Verification items for this drawing (mm, ordinates from the low corner). Coordinates: 2 decimals unless noted, no trailing zeros. Write each loop counter-clockwise with the first axis right and the second up, starting at its lowest first coordinate (ties: lowest second). Pieces come first, ordered by that corner, then holes. Notation, with made-up numbers: M 64,72 L 80,72 A17 cw 80,82 Z; hole C 23.25,71.25 d9. An arc over 180 degrees is marked long. Answer as CSV lines item,"result". Start each with the question number.
1) Material ranges on L1, parallel to Y at x = 7.75, z = 19.05 (1 decimal); L2, parallel to Z at x = 9.5, y = 11.5 (1 decimal); L3, parallel to Z at x = 11.5, y = 19.05 (1 decimal), recorded low to high. Write a range as [from, to].
2) Section check B-B (y = 19.05). Record the cut outline in (x, z) (1 decimal).
3) Draft check along Y on the marked faces 1, 2 and 3. Enter one of: +Y half, -Y half, draft (parallel to the pull), parting line (faces both ways), or undercut.
4) Go/stop test with flat-tipped pins: pin 1 Ø10 at (y, z) = (13.97, 10.25) entering from +X; pin 2 Ø5.5 at (y, z) = (13.97, 27.85) entering from +X; pin 3 Ø3 at (x, z) = (4.5, 33) entering from -Y; pin 4 Ø5 at (x, y) = (9, 32.5) entering from +Z (1 decimal). Record where each tip stops, or that it passes through.
5) Section check A-A (z = 19.05). Record the cut outline in (x, y) (1 decimal).
6) Section check C-C (x = 8). State how many separate pieces and enclosed holes the cut face has, and give its area (3 significant figures).
7) Section check D-D (y = 13.97). Record the cut outline in (x, z) (1 decimal), and give its area (3 significant figures).
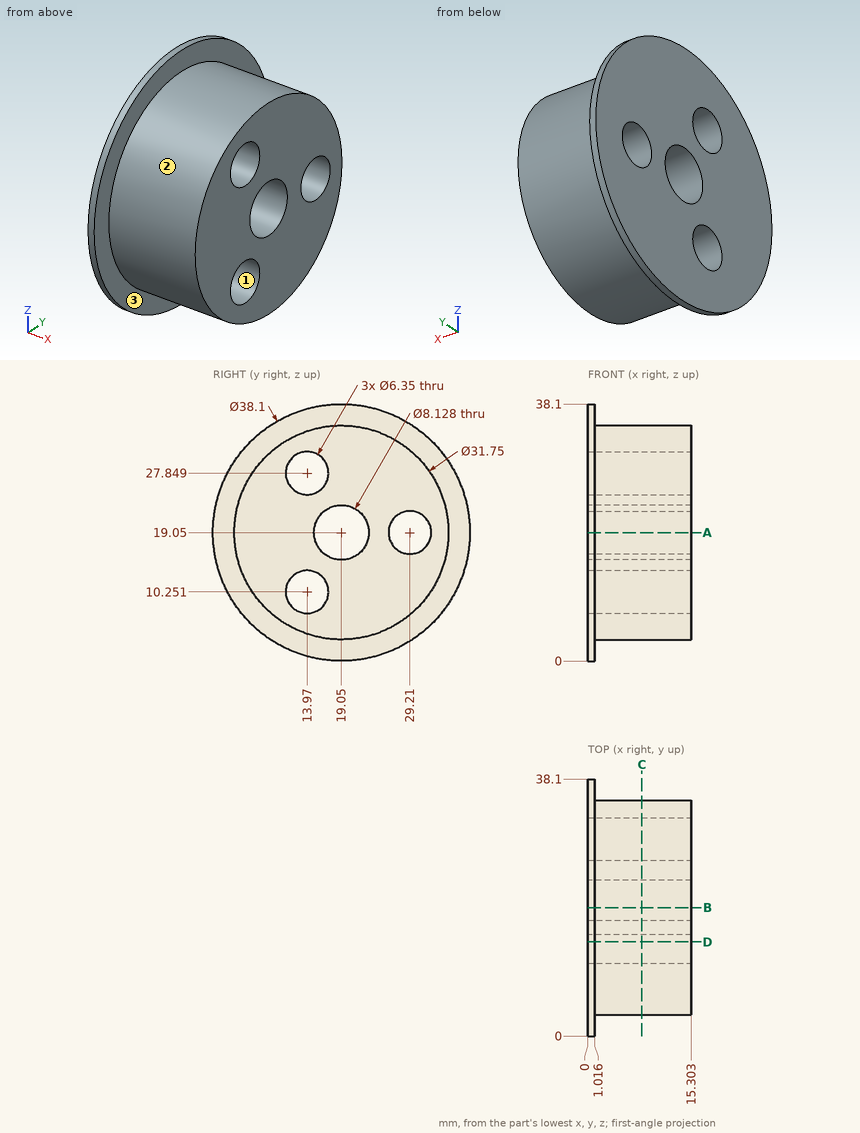
Results found:
1,L1,"y = [3.2, 15], [23.1, 26], [32.4, 34.9]"
1,L2,"z = [5.1, 8.3], [12.2, 25.9], [29.8, 33]"
1,L3,"z = [3.2, 15], [23.1, 34.9]"
2,outline,"M 0,0 L 1,0 L 1,3.2 L 15.3,3.2 L 15.3,15 L 0,15 Z; M 0,23.1 L 15.3,23.1 L 15.3,34.9 L 1,34.9 L 1,38.1 L 0,38.1 Z"
3,face 1,"undercut"
3,face 2,"parting line"
3,face 3,"draft"
4,pin 1,"stops at x = 15.3"
4,pin 2,"passes through"
4,pin 3,"stops at y = 9.2"
4,pin 4,"stops at z = 30.5"
5,outline,"M 0,0 L 1,0 L 1,3.2 L 15.3,3.2 L 15.3,15 L 0,15 Z; M 0,23.1 L 15.3,23.1 L 15.3,26 L 0,26 Z; M 0,32.4 L 15.3,32.4 L 15.3,34.9 L 1,34.9 L 1,38.1 L 0,38.1 Z"
6,separate pieces,"1"
6,enclosed holes,"4"
6,area,"645 mm2"
7,outline,"M 0,0.7 L 1,0.7 L 1,4 L 15.3,4 L 15.3,7.1 L 0,7.1 Z; M 0,13.4 L 15.3,13.4 L 15.3,24.7 L 0,24.7 Z; M 0,31 L 15.3,31 L 15.3,34.1 L 1,34.1 L 1,37.4 L 0,37.4 Z"
7,area,"273 mm2"
